```python
from build123d import *

# Parameters (mm, degrees)
BOSS_EXTRUDE1_DEPTH = 22.225
SKETCH8_R           = 3.175
CUT_EXTRUDE7_DEPTH  = 29.21
CUT_EXTRUDE8_REACH  = 75.025


with BuildPart() as part:
    # Sketch1 → Boss-Extrude1 (new body)
    with BuildSketch(Plane.XY):
        Polygon((0, 0), (0, 22.225), (53.975, 22.225), (53.975, 20.6375), (73.025, 1.5875), (73.025, 0), align=None)
    extrude(amount=BOSS_EXTRUDE1_DEPTH)

    # Sketch8 → Cut-Extrude7 (cut)
    with BuildSketch(Plane.XY.offset(22.225)):
        with Locations((9.525, 11.1125)):
            Circle(SKETCH8_R)
        with BuildLine():
            Line((22.225, 14.2875), (47.625, 14.2875))
            ThreePointArc((47.625, 14.2875), (50.8, 11.1125), (47.625, 7.9375))
            Line((47.625, 7.9375), (22.225, 7.9375))
            ThreePointArc((22.225, 7.9375), (19.05, 11.1125), (22.225, 14.2875))
        make_face()
    extrude(amount=-CUT_EXTRUDE7_DEPTH, mode=Mode.SUBTRACT)

    # Sketch10 → Cut-Extrude8 (cut, up to next)
    with BuildSketch(Plane.ZY, mode=Mode.PRIVATE) as cut_extrude8_sk1:
        with BuildLine():
            Line((3.175, 14.2875), (0, 14.2875))
            Line((0, 14.2875), (0, 7.9375))
            Line((0, 7.9375), (3.175, 7.9375))
            ThreePointArc((3.175, 7.9375), (6.35, 11.1125), (3.175, 14.2875))
        make_face()
    cut_extrude8_tool1 = extrude(cut_extrude8_sk1.sketch, amount=-CUT_EXTRUDE8_REACH, mode=Mode.PRIVATE) & part.part
    add(cut_extrude8_tool1.solids().sort_by_distance((0, 11.1125, 2.878614))[0], mode=Mode.SUBTRACT)
    # Sketch10 → Cut-Extrude8 (cut, up to next)
    with BuildSketch(Plane.ZY, mode=Mode.PRIVATE) as cut_extrude8_sk2:
        with BuildLine():
            Line((19.05, 7.9375), (22.225, 7.9375))
            Line((22.225, 7.9375), (22.225, 14.2875))
            Line((22.225, 14.2875), (19.05, 14.2875))
            ThreePointArc((19.05, 14.2875), (15.875, 11.1125), (19.05, 7.9375))
        make_face()
    cut_extrude8_tool2 = extrude(cut_extrude8_sk2.sketch, amount=-CUT_EXTRUDE8_REACH, mode=Mode.PRIVATE) & part.part
    add(cut_extrude8_tool2.solids().sort_by_distance((0, 11.1125, 19.346386))[0], mode=Mode.SUBTRACT)


solid = part.part
```
CAD build for the part. Positions are in the model's coordinates, mm. A direction names the side the tool comes from. Round coordinates to 2 decimals unless told otherwise and drop trailing zeros. Loops run counter-clockwise (first coordinate to the right, second up) from the corner with the lowest first, then second, coordinate; pieces in that order, holes last. Notation, with made-up numbers: M -14.75,-1 L 43.25,-1 A24 cw 43.25,15 Z; hole C 5.5,67 d2. An arc over 180 degrees is marked long. Use a Markdown table: item, result. Add a question column.
(1) Flat gauge pin, fed straight in: pin 1 (8 mm diameter, centred on y = 16, z = 3, fed in from +X). Where does the tip first touch, or does it go through?
(2) Which spindle directions (+Z, -Z, +X, -X, +Y, -Y) get a long thin tool onto all of the face, cutting with end or side? Do faces 4 (the face through (53.975, 21, 11)), 5 (the face through (5, 14.288, 2)), 6 (the face through (5, 7.938, 21)), 7 (the face through (19.05, 11.04, 11.27)), 8 (the face through (37, 0, 11)). Say none if no direction does.
(3) Cut at D-D (x = 62.5). Give the cut face in (y, z) (1 decimal), and give its area (3 significant figures).
(4) Cut at C-C (y = 15). Give the cut face in (x, z) (1 decimal), and give its area (3 significant figures).
(5) Pull direction Y, two halves, no side cores. Call faces 1 (the face through (63.367, 11.246, 10.957)), 2 (the face through (37, 6, 22.225)), 3 (the face through (50.8, 11.2, 11.3)): +Y half, -Y half, draft (parallel to the pull), parting line (faces both ways), or undercut.
(6) Drill centre lines: line 1 (Y direction, x = 35.5, z = 17.75) (1 decimal); line 2 (X direction, y = 13.5, z = 7.25); line 3 (X direction, y = 9.5, z = 6.75). Where is each one in solid material? Low to high.
Geometry says:
| question | item | result |
|---|---|---|
| 1 | pin 1 | stops at x = 62.61 |
| 2 | face 4 | +Z, -Z, +X, +Y |
| 2 | face 5 | -Z, -X |
| 2 | face 6 | +Z, -X |
| 2 | face 7 | +Z, -Z |
| 2 | face 8 | +Z, -Z, +X, -X, -Y |
| 3 | outline | M 0,0 L 12.1,0 L 12.1,22.2 L 0,22.2 Z |
| 3 | area | 269 mm² |
| 4 | outline | M 0,0 L 59.6,0 L 59.6,22.2 L 0,22.2 Z |
| 4 | area | 1,320 mm² |
| 5 | face 1 | +Y half |
| 5 | face 2 | draft |
| 5 | face 3 | undercut |
| 6 | line 1 | y = 0 to 7.9, 14.3 to 22.2 |
| 6 | line 2 | x = 0 to 7.43, 11.62 to 20.13, 49.72 to 61.11 |
| 6 | line 3 | x = 0 to 6.79, 12.26 to 19.49, 50.36 to 65.11 |
